Source: CAD feature listing. Evaluate the final solid. Frame: model axes, mm. A direction names the side the tool comes from. Give positions to 0.01 mm unless a question says otherwise; leave off trailing zeros. Loops run counter-clockwise (first coordinate to the right, second up) from the corner with the lowest first, then second, coordinate; pieces in that order, holes last. Notation, with made-up numbers: M -11,-36.5 L -2,-36.5 A34 cw -2,-0.5 Z; hole C 20,-17.5 d3. An arc over 180 degrees is marked long. Answer in a Markdown table with one row per item.
```python
from build123d import *

# Parameters (mm, degrees)
SKIZZE1_W                       = 48
SKIZZE1_H                       = 48
AUFSATZ_LINEAR_AUSTRAGEN1_DEPTH = 4
SKIZZE2_W                       = 5
SKIZZE2_H                       = 10
SKIZZE2_W_2                     = 15
SKIZZE2_H_2                     = 5
AUFSATZ_LINEAR_AUSTRAGEN3_DEPTH = 10
FASE1_SIZE                      = 10
SCHNITT_LINEAR_AUSTRAGEN1_REACH = 68.603
SKIZZE3_R                       = 1
SCHNITT_LINEAR_AUSTRAGEN2_REACH = 68.603
SKIZZE4_R                       = 1
SCHNITT_LINEAR_AUSTRAGEN3_REACH = 70.615
SKIZZE5_R                       = 1.5


with BuildPart() as part:
    # Skizze1 → Aufsatz-Linear austragen1 (new body)
    with BuildSketch(Plane.XY):
        with Locations((24, 24)):
            Rectangle(SKIZZE1_W, SKIZZE1_H)
    extrude(amount=AUFSATZ_LINEAR_AUSTRAGEN1_DEPTH)

    # Skizze2 → Aufsatz-Linear austragen3 (add)
    with BuildSketch(Plane.XY.offset(4)):
        with Locations((6.5, 34)):
            Rectangle(SKIZZE2_W, SKIZZE2_H)
        with Locations((11.5, 41.5)):
            Rectangle(SKIZZE2_W_2, SKIZZE2_H_2)
        with Locations((36.5, 41.5)):
            Rectangle(SKIZZE2_W_2, SKIZZE2_H_2)
        with Locations((41.5, 34)):
            Rectangle(SKIZZE2_W, SKIZZE2_H)
        with Locations((41.5, 14)):
            Rectangle(SKIZZE2_W, SKIZZE2_H)
        with Locations((36.5, 6.5)):
            Rectangle(SKIZZE2_W_2, SKIZZE2_H_2)
        with Locations((11.5, 6.5)):
            Rectangle(SKIZZE2_W_2, SKIZZE2_H_2)
        with Locations((6.5, 14)):
            Rectangle(SKIZZE2_W, SKIZZE2_H)
    extrude(amount=AUFSATZ_LINEAR_AUSTRAGEN3_DEPTH)

    # Fase1
    fase1_edges = [part.edges().sort_by_distance(p)[0] for p in [
        (19, 41.5, 14),
        (29, 41.5, 14),
        (41.5, 29, 14),
        (41.5, 19, 14),
        (29, 6.5, 14),
        (6.5, 19, 14),
        (6.5, 29, 14),
        (19, 6.5, 14),
    ]]
    chamfer(fase1_edges, length=FASE1_SIZE - 0.0001)  # a hair under: the kernel refuses the full size

    # Schnitt-Linear austragen1: up to this face of the body (flat: up to its plane)
    schnitt_linear_austragen1_end = Plane(part.part.faces().sort_by_distance((9.4167125, 44, 8.166675))[0])
    # Skizze3 → Schnitt-Linear austragen1 (cut, up to the picked face)
    with BuildSketch(Plane.XZ.offset(-4), mode=Mode.PRIVATE) as schnitt_linear_austragen1_sk1:
        with Locations(Location((9, 9, 0), (0, 0, 90))):
            Circle(SKIZZE3_R)
    schnitt_linear_austragen1_tool1 = split(extrude(schnitt_linear_austragen1_sk1.sketch, amount=-SCHNITT_LINEAR_AUSTRAGEN1_REACH, mode=Mode.PRIVATE), bisect_by=schnitt_linear_austragen1_end, keep=Keep.BOTH, mode=Mode.PRIVATE)
    # Skizze3 → Schnitt-Linear austragen1 (cut, up to the picked face)
    with BuildSketch(Plane.XZ.offset(-4), mode=Mode.PRIVATE) as schnitt_linear_austragen1_sk2:
        with Locations((39, 9)):
            Circle(SKIZZE3_R)
    schnitt_linear_austragen1_tool2 = split(extrude(schnitt_linear_austragen1_sk2.sketch, amount=-SCHNITT_LINEAR_AUSTRAGEN1_REACH, mode=Mode.PRIVATE), bisect_by=schnitt_linear_austragen1_end, keep=Keep.BOTH, mode=Mode.PRIVATE)
    add(schnitt_linear_austragen1_tool1.solids().sort_by(Axis((9, 4, 9), (0, 1, 0)))[0], mode=Mode.SUBTRACT)
    add(schnitt_linear_austragen1_tool2.solids().sort_by(Axis((39, 4, 9), (0, 1, 0)))[0], mode=Mode.SUBTRACT)

    # Schnitt-Linear austragen2: up to this face of the body (flat: up to its plane)
    schnitt_linear_austragen2_end = Plane(part.part.faces().sort_by_distance((44, 9.4167125, 8.166675))[0])
    # Skizze4 → Schnitt-Linear austragen2 (cut, up to the picked face)
    with BuildSketch(Plane.ZY.offset(-4), mode=Mode.PRIVATE) as schnitt_linear_austragen2_sk1:
        with Locations(Location((9, 39, 0), (0, 0, 180))):
            Circle(SKIZZE4_R)
    schnitt_linear_austragen2_tool1 = split(extrude(schnitt_linear_austragen2_sk1.sketch, amount=-SCHNITT_LINEAR_AUSTRAGEN2_REACH, mode=Mode.PRIVATE), bisect_by=schnitt_linear_austragen2_end, keep=Keep.BOTH, mode=Mode.PRIVATE)
    # Skizze4 → Schnitt-Linear austragen2 (cut, up to the picked face)
    with BuildSketch(Plane.ZY.offset(-4), mode=Mode.PRIVATE) as schnitt_linear_austragen2_sk2:
        with Locations(Location((9, 9, 0), (0, 0, 180))):
            Circle(SKIZZE4_R)
    schnitt_linear_austragen2_tool2 = split(extrude(schnitt_linear_austragen2_sk2.sketch, amount=-SCHNITT_LINEAR_AUSTRAGEN2_REACH, mode=Mode.PRIVATE), bisect_by=schnitt_linear_austragen2_end, keep=Keep.BOTH, mode=Mode.PRIVATE)
    add(schnitt_linear_austragen2_tool1.solids().sort_by(Axis((4, 39, 9), (1, 0, 0)))[0], mode=Mode.SUBTRACT)
    add(schnitt_linear_austragen2_tool2.solids().sort_by(Axis((4, 9, 9), (1, 0, 0)))[0], mode=Mode.SUBTRACT)

    # Skizze5 → Schnitt-Linear austragen3 (cut, up to next)
    with BuildSketch(Plane.XY.offset(4), mode=Mode.PRIVATE) as schnitt_linear_austragen3_sk1:
        with Locations((34, 14)):
            Circle(SKIZZE5_R)
    schnitt_linear_austragen3_tool1 = extrude(schnitt_linear_austragen3_sk1.sketch, amount=-SCHNITT_LINEAR_AUSTRAGEN3_REACH, mode=Mode.PRIVATE) & part.part
    # Skizze5 → Schnitt-Linear austragen3 (cut, up to next)
    with BuildSketch(Plane.XY.offset(4), mode=Mode.PRIVATE) as schnitt_linear_austragen3_sk2:
        with Locations((14, 14)):
            Circle(SKIZZE5_R)
    schnitt_linear_austragen3_tool2 = extrude(schnitt_linear_austragen3_sk2.sketch, amount=-SCHNITT_LINEAR_AUSTRAGEN3_REACH, mode=Mode.PRIVATE) & part.part
    # Skizze5 → Schnitt-Linear austragen3 (cut, up to next)
    with BuildSketch(Plane.XY.offset(4), mode=Mode.PRIVATE) as schnitt_linear_austragen3_sk3:
        with Locations((14, 34)):
            Circle(SKIZZE5_R)
    schnitt_linear_austragen3_tool3 = extrude(schnitt_linear_austragen3_sk3.sketch, amount=-SCHNITT_LINEAR_AUSTRAGEN3_REACH, mode=Mode.PRIVATE) & part.part
    # Skizze5 → Schnitt-Linear austragen3 (cut, up to next)
    with BuildSketch(Plane.XY.offset(4), mode=Mode.PRIVATE) as schnitt_linear_austragen3_sk4:
        with Locations((34, 34)):
            Circle(SKIZZE5_R)
    schnitt_linear_austragen3_tool4 = extrude(schnitt_linear_austragen3_sk4.sketch, amount=-SCHNITT_LINEAR_AUSTRAGEN3_REACH, mode=Mode.PRIVATE) & part.part
    add(schnitt_linear_austragen3_tool1.solids().sort_by_distance((34, 14, 4))[0], mode=Mode.SUBTRACT)
    add(schnitt_linear_austragen3_tool2.solids().sort_by_distance((14, 14, 4))[0], mode=Mode.SUBTRACT)
    add(schnitt_linear_austragen3_tool3.solids().sort_by_distance((14, 34, 4))[0], mode=Mode.SUBTRACT)
    add(schnitt_linear_austragen3_tool4.solids().sort_by_distance((34, 34, 4))[0], mode=Mode.SUBTRACT)


solid = part.part
```
Q1. Mould query, pull axis Y, two halves, no side actions, for faces 1 (the flat face through (24, 48, 2)), 2 (the cylindrical face through (8, 6, 9)), 3 (the flat face through (6, 14, 9)). Classes: +Y half, -Y half, draft (parallel to the pull), parting line (faces both ways), or undercut.
Values follow:
| item | result |
|---|---|
| face 1 | +Y half |
| face 2 | draft |
| face 3 | undercut |
Q2. Section query B-B (x = 42). Give the number of separate pieces and of enclosed holes in the cut face, plus the area to 3 significant figures.
Values follow:
| item | result |
|---|---|
| separate pieces | 1 |
| enclosed holes | 2 |
| area | 386 mm^2 |
Q3. Section query C-C (z = 11.5). Output: boundary loops of the cut face in (x, y).
Values follow:
| item | result |
|---|---|
| outline | M 4,4 L 11.5,4 L 11.5,9 L 9,9 L 9,11.5 L 4,11.5 Z; M 4,36.5 L 9,36.5 L 9,39 L 11.5,39 L 11.5,44 L 4,44 Z; M 36.5,4 L 44,4 L 44,11.5 L 39,11.5 L 39,9 L 36.5,9 Z; M 36.5,39 L 39,39 L 39,36.5 L 44,36.5 L 44,44 L 36.5,44 Z |
Q4. Section query A-A (x = 14). Output: boundary loops of the cut face in (y, z), plus the area to 3 significant figures.
Values follow:
| item | result |
|---|---|
| outline | M 0,0 L 12.5,0 L 12.5,4 L 9,4 L 9,8 A1 cw 8,9 L 4,9 L 4,4 L 0,4 Z; M 15.5,0 L 32.5,0 L 32.5,4 L 15.5,4 Z; M 35.5,0 L 48,0 L 48,4 L 44,4 L 44,9 L 40,9 A1 cw 39,8 L 39,4 L 35.5,4 Z |
| area | 216 mm^2 |
Q5. Section query D-D (y = 30). Output: boundary loops of the cut face in (x, z), plus the area to 3 significant figures.
Values follow:
| item | result |
|---|---|
| outline | M 0,0 L 48,0 L 48,4 L 44,4 L 44,5 L 39,5 L 39,4 L 9,4 L 9,5 L 4,5 L 4,4 L 0,4 Z |
| area | 202 mm^2 |
Q6. Contact query for flat-ended pins moving along their axis: pin 1 Ø1.5 at (x, y) = (19, 12.5) entering from +Z; pin 2 Ø1.5 at (y, z) = (37, 11) entering from +X; pin 3 Ø2 at (x, z) = (11.5, 12.5) entering from -Y. Output: stop coordinate, or through.
Values follow:
| item | result |
|---|---|
| pin 1 | z = 4 |
| pin 2 | x = 44 |
| pin 3 | y = 4 |
Q7. Ray query, probe 1 along Y at (x, z) = (34, 2.1); probe 2 along Y at (x, z) = (35, 7.75); probe 3 along Z at (x, y) = (5.3, 39). Return the intervals inside material, ascending. Write a range as from..to.
Values follow:
| item | result |
|---|---|
| probe 1 | 0..12.5, 15.5..32.5, 35.5..48 |
| probe 2 | 4..9, 39..44 |
| probe 3 | 0..8, 10..14 |
Q8. Reachability of faces 4 (the cylindrical face through (8, 12, 9)), 5 (the flat face through (24, 24, 4)), 6 (the flat face through (10, 44, 8)) from +Z, -Z, +X, -X, +Y, -Y: full face, straight path, thin tool, end or side. Return the list, or none.
Values follow:
| item | result |
|---|---|
| face 4 | +Y, -Y |
| face 5 | +Z |
| face 6 | +Z, +X, -X, +Y |
